Here's the drawing with two shaded views (mm, measured from the low corner). I have some questions. Coordinates: 2 decimals unless noted, no trailing zeros. Write each loop counter-clockwise with the first axis right and the second up, starting at its lowest first coordinate (ties: lowest second). Pieces come first, ordered by that corner, then holes. Notation, with made-up numbers: (33, 2.5) - (90, 2.5) arc R20 cw to (90, 28.5) - close; hole circle Ø11 at (37, 31). An arc over 180 degrees is marked (long way). Answer in a Markdown table with one row per item. Add a question column.
Item 1: Imagine slicing it at A-A (z = 25.4). Please give me the cut outline in (x, y) (3 decimals), plus the area to 3 significant figures.
Item 2: Imagine slicing it at B-B (x = 53.5). Please give me the cut outline in (y, z), plus the area to 3 significant figures.
Item 3: If I drill on probe 1 along X at (y, z) = (1.5, 25.4) (3 decimals); probe 2 along X at (y, z) = (1.8, 44.5); probe 3 along Z at (x, y) = (41.5, 2.7), over which ranges is the centre line in solid material (lowest first)? Write a range as from..to.
Item 4: Imagine slicing it at C-C (y = 0.65). Please give me the cut outline in (x, z) (3 decimals).
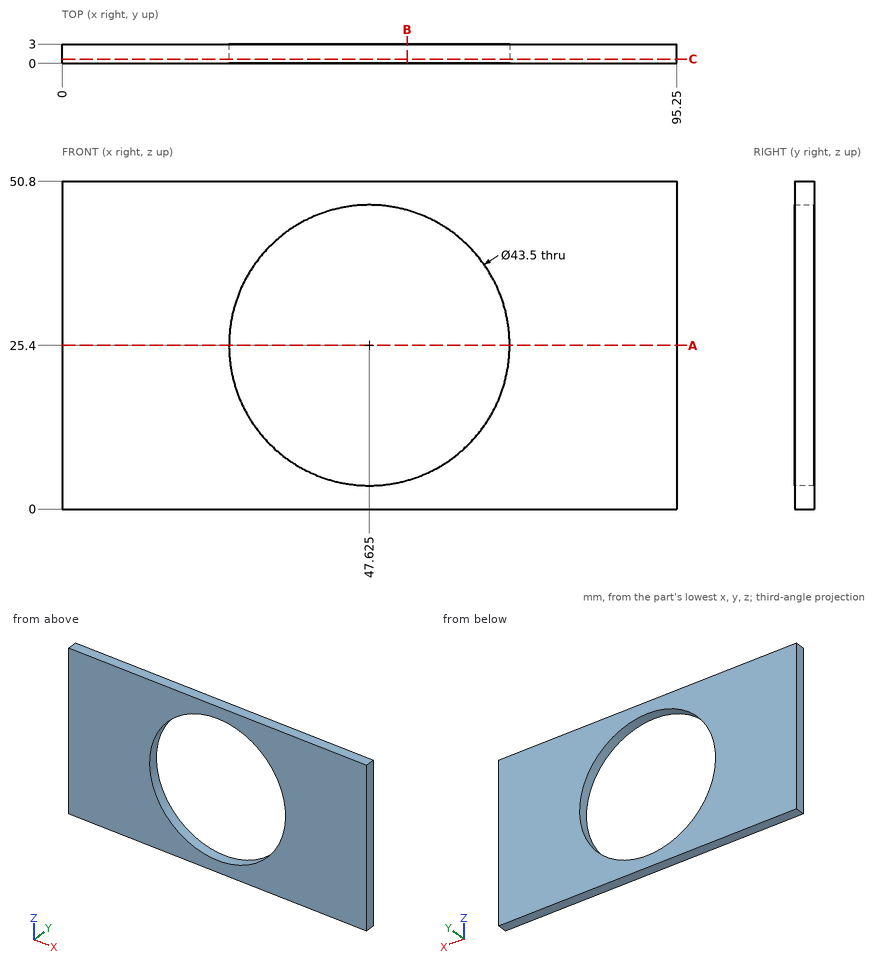
Here are the results:
| question | item | result |
|---|---|---|
| 1 | outline | (0, 0) - (25.875, 0) - (25.875, 3) - (0, 3) - close; (69.375, 0) - (95.25, 0) - (95.25, 3) - (69.375, 3) - close |
| 1 | area | 155 mm2 |
| 2 | outline | (0, 0) - (3, 0) - (3, 4.46) - (0, 4.46) - close; (0, 46.34) - (3, 46.34) - (3, 50.8) - (0, 50.8) - close |
| 2 | area | 26.8 mm2 |
| 3 | probe 1 | x = 0..25.875, 69.375..95.25 |
| 3 | probe 2 | x = 0..37.22, 58.03..95.25 |
| 3 | probe 3 | z = 0..4.53, 46.27..50.8 |
| 4 | outline | (0, 0) - (95.25, 0) - (95.25, 50.8) - (0, 50.8) - close; hole circle Ø43.5 at (47.625, 25.4) |
